```python
from build123d import *

# Parameters (mm, degrees)
SKETCH1_R               = 64.345413168
BOSS_EXTRUDE1_DEPTH     = 40
SKETCH3_R               = 14.331573803
CUT_EXTRUDE2_DEPTH      = 40
CUT_EXTRUDE3_DEPTH      = 179.175578552
CUT_EXTRUDE3_DEPTH_BACK = 40
SKETCH5_R               = 17.792090532
CUT_EXTRUDE6_DEPTH      = 18


with BuildPart() as part:
    # Sketch1 → Boss-Extrude1 (new body)
    with BuildSketch(Plane.XY):
        with Locations((-96.918980287, 0)):
            Circle(SKETCH1_R)
    extrude(amount=BOSS_EXTRUDE1_DEPTH)

    # Sketch3 → Cut-Extrude2 (cut)
    with BuildSketch(Plane.XY.offset(40)):
        with Locations((-95.729315352, 0)):
            Circle(SKETCH3_R)
    extrude(amount=-CUT_EXTRUDE2_DEPTH, mode=Mode.SUBTRACT)

    # Sketch4 → Cut-Extrude3 (cut, two sides: drawn at the far end of the back side and taken through both)
    with BuildSketch(Plane.XY.offset(40).offset(-CUT_EXTRUDE3_DEPTH_BACK)):
        Polygon((268.087714355, 281.481110593), (-21.116990888, 49.302685257), (-148.180972854, -52.706427026), (-437.385678097, -284.884852362), (26.971172575, -863.294262848), (732.444565027, -296.928299893), align=None)
    extrude(amount=CUT_EXTRUDE3_DEPTH + CUT_EXTRUDE3_DEPTH_BACK, mode=Mode.SUBTRACT)

    # Sketch5 → Cut-Extrude6 (cut)
    with BuildSketch(Plane(origin=(-32.344640606, 40.288938299, 0), x_dir=(0.7797961442184731, 0.626033524231732, 0), z_dir=(0.626033524231732, -0.7797961442184731, 0))):
        with Locations((-34.092669142, 19.900069025)):
            Circle(SKETCH5_R)
    extrude(amount=-CUT_EXTRUDE6_DEPTH, mode=Mode.SUBTRACT)


solid = part.part
```
Here's how the part is built. I have some questions about the finished solid (model axes, mm). A direction names the side the tool comes from. Coordinates: 2 decimals unless noted, no trailing zeros. Write each loop counter-clockwise with the first axis right and the second up, starting at its lowest first coordinate (ties: lowest second). Pieces come first, ordered by that corner, then holes. Notation, with made-up numbers: (4, 7.5) -> (27, 7.5) arc R25 cw to (27, 31.5) -> close; hole circle Ø5 at (-32, 34.25). An arc over 180 degrees is marked (long way). Use a Markdown table: item, result. Add a question column.
(1) If we section it at A-A, the plane z = 31: Write out the boundary of the cut face in (x, y), and give its area (3 significant figures).
(2) I'm going to push flat-ended pins straight in: P1, Ø5, axis at y = -0.5, z = 13.5, coming from the +X side; P2, Ø4, axis at y = 10, z = 6, coming from the +X side; P3, Ø6, axis at y = 41.5, z = 26, coming from the +X side; P4, Ø12, axis at x = -134, y = -29.5, coming from the -Z side. Where does each tip first touch, or does it pass through?
(3) For faces 1 (the flat face through (-70.39, 32.83, 20.15)), 2 (the flat face through (-116, 22, 0)), which set-ups out of +Z, -Z, +X, -X, +Y, -Y let a thin tool reach every point of the face, with its end or its side?
(4) If we section it at C-C, the plane z = 18: Write out the boundary of the cut face in (x, y).
(5) If we section it at D-D, the plane x = -130.5: Write out the boundary of the cut face in (y, z).
(6) If we section it at B-B, the plane y = -15.5: Write out the boundary of the cut face in (x, z).
(7) Please list where these lines run through material, in increasing order: line 1 (X direction, y = 0, z = 30); line 2 (Y direction, x = -77.5, z = 8.5); line 3 (X direction, y = 1, z = 17).
(8) We'd pull the mould along X, two halves only. Please class faces 3 (the cylindrical face through (-51.7, 36.2, 13.1)), 4 (the cylindrical face through (-104.36, 11.44, 20.28)), 5 (the cylindrical face through (-135.988, 51.127, 19.72)), 6 (the flat face through (-120.035, -30.11, 19.72)): +X half, -X half, draft (parallel to the pull), parting line (faces both ways), or undercut.
Outcome:
| question | item | result |
|---|---|---|
| 1 | outline | (-140.96, -46.91) -> (-99.69, -13.77) arc R14.33 cw (long way) to (-81.43, 0.89) -> (-69.77, 10.24) -> (-81.04, 24.28) -> (-59.36, 41.69) -> (-48.09, 27.65) -> (-41.6, 32.86) arc R64.35 ccw (long way) to start |
| 1 | area | 6,610 mm^2 |
| 2 | P1 | stops at x = -80.04 |
| 2 | P2 | stops at x = -67.58 |
| 2 | P3 | stops at x = -45.36 |
| 2 | P4 | stops at z = 0 |
| 3 | face 1 | none |
| 3 | face 2 | -Z, +X, -X, +Y, -Y |
| 4 | outline | (-140.96, -46.91) -> (-99.69, -13.77) arc R14.33 cw (long way) to (-81.43, 0.89) -> (-72.72, 7.87) -> (-83.99, 21.91) -> (-56.4, 44.06) -> (-45.14, 30.02) -> (-41.6, 32.86) arc R64.35 ccw (long way) to start |
| 5 | outline | (-38.51, 0) -> (54.89, 0) -> (54.89, 40) -> (-38.51, 40) -> close |
| 6 | outline | (-159.37, 0) -> (-101.84, 0) -> (-101.84, 40) -> (-159.37, 40) -> close |
| 7 | line 1 | x = -161.26 to -110.06 |
| 7 | line 2 | y = 4.04 to 20.26, 27.12 to 61.35 |
| 7 | line 3 | x = -161.26 to -110.03, -81.43 to -81.28 |
| 8 | face 3 | undercut |
| 8 | face 4 | undercut |
| 8 | face 5 | parting line |
| 8 | face 6 | +X half |
